Verification items for the finished model (mm, model axes). Coordinates: 2 decimals unless noted, no trailing zeros. Loops run counter-clockwise (first coordinate to the right, second up) from the corner with the lowest first, then second, coordinate; pieces in that order, holes last. Notation, with made-up numbers: (81, -7) -> (127, -7) arc R33 cw to (127, 23) -> close; hole circle Ø10 at (-6, -18.5). An arc over 180 degrees is marked (long way). Write item = value, one per line.
```python
from build123d import *

# Parameters (mm, degrees)
BOSS_EXTRUDE1_DEPTH = 6
SKETCH2_W           = 6
SKETCH2_H           = 37.5
CUT_EXTRUDE1_DEPTH  = 6
LPATTERN1_COUNT     = 4
LPATTERN1_PITCH     = 75
FILLET1_R           = 40
SKETCH3_W           = 6
SKETCH3_H           = 10
SKETCH3_H_2         = 112.5
CUT_EXTRUDE2_DEPTH  = 515.816472153
SKETCH4_W           = 15
SKETCH4_H           = 6
CUT_EXTRUDE3_DEPTH  = 515.816472153
SKETCH5_R           = 2
CUT_EXTRUDE4_DEPTH  = 515.816472153


with BuildPart() as part:
    # Sketch1 → Boss-Extrude1 (new body)
    with BuildSketch(Plane(origin=(0, 0, 0), x_dir=(0, 0, -1), z_dir=(1, 0, 0))):
        Polygon((450, 225), (450, 250), (0, 250), (0, 0), (450, 0), (450, 127.5), (30, 127.5), (30, 225), align=None)
    extrude(amount=BOSS_EXTRUDE1_DEPTH)

    # Sketch2 → Cut-Extrude1 (cut)
    with BuildSketch(Plane(origin=(6, 0, 0), x_dir=(0, 0, -1), z_dir=(1, 0, 0))):
        with Locations((3, 231.25)):
            Rectangle(SKETCH2_W, SKETCH2_H)
    cut_extrude1 = extrude(amount=-CUT_EXTRUDE1_DEPTH, mode=Mode.SUBTRACT)

    # LPattern1: Cut-Extrude1 ×4
    with Locations(*[(0, -i * LPATTERN1_PITCH, 0) for i in range(1, LPATTERN1_COUNT)]):
        add(cut_extrude1, mode=Mode.SUBTRACT)

    # Fillet1
    fillet1_edges = [part.edges().sort_by_distance(p)[0] for p in [
        (3, 225, -30),
    ]]
    fillet(fillet1_edges, radius=FILLET1_R)

    # Sketch3 → Cut-Extrude2 (cut, through all)
    with BuildSketch(Plane.ZY):
        with Locations((-447, 230)):
            Rectangle(SKETCH3_W, SKETCH3_H)
        with Locations((-447, 56.25)):
            Rectangle(SKETCH3_W, SKETCH3_H_2)
    extrude(amount=-CUT_EXTRUDE2_DEPTH, mode=Mode.SUBTRACT)

    # Sketch4 → Cut-Extrude3 (cut, through all)
    with BuildSketch(Plane.ZY):
        with Locations((-23.5, 3)):
            Rectangle(SKETCH4_W, SKETCH4_H)
        with Locations((-426.5, 3)):
            Rectangle(SKETCH4_W, SKETCH4_H)
    extrude(amount=-CUT_EXTRUDE3_DEPTH, mode=Mode.SUBTRACT)

    # Sketch5 → Cut-Extrude4 (cut, through all)
    with BuildSketch(Plane.ZY):
        with Locations((-384, 237.5)):
            Circle(SKETCH5_R)
        with Locations((-364, 237.5)):
            Circle(SKETCH5_R)
    extrude(amount=-CUT_EXTRUDE4_DEPTH, mode=Mode.SUBTRACT)


solid = part.part
```
1) Depth check by flat-ended pin: pin 1 Ø1.8 at (x, z) = (3, -2.5) entering from +Y; pin 2 Ø1.5 at (x, y) = (4.5, 161.5) entering from +Z; pin 3 Ø3 at (x, y) = (4.5, 4.5) entering from -Z; pin 4 Ø3.5 at (y, z) = (237.5, -364) entering from -X. Enter the tip coordinate at first touch or a pass-through.
Ans:
pin_1 = 212.5
pin_2 = -6
pin_3 = -444
pin_4 = through
2) Sectioned sample at C-C, the plane z = -44.5. Record the cut outline in (x, y), plus the area to 3 significant figures.
Ans:
outline = (0, 0) -> (6, 0) -> (6, 127.5) -> (0, 127.5) -> close; (0, 215.82) -> (6, 215.82) -> (6, 250) -> (0, 250) -> close
area = 970 mm2
3) Sectioned sample at A-A, the plane z = -177.5. Record the cut outline in (x, y).
Ans:
outline = (0, 0) -> (6, 0) -> (6, 127.5) -> (0, 127.5) -> close; (0, 225) -> (6, 225) -> (6, 250) -> (0, 250) -> close
4) Material ranges on line 1 (Y direction, x = 4.6, z = -364); line 2 (Z direction, x = 2.2, y = 237.5); line 3 (Y direction, x = 1.75, z = -224.5), recorded low to high.
Ans:
line_1 = 0 to 127.5, 225 to 235.5, 239.5 to 250
line_2 = -450 to -386, -382 to -366, -362 to -6
line_3 = 0 to 127.5, 225 to 250
5) Sectioned sample at D-D, the plane y = 164.5. Record the cut outline in (x, z), plus the area to 3 significant figures.
Ans:
outline = (0, -30) -> (6, -30) -> (6, -6) -> (0, -6) -> close
area = 144 mm2
6) Sectioned sample at B-B, the plane x = 2.75. Count the separate pieces of the cut face and the enclosed holes in it, plus the area to 3 significant figures.
Ans:
separate_pieces = 1
enclosed_holes = 2
area = 70,100 mm2
7) Release check for a two-part mould opening along Y. For faces 1 (the face through (3.042, 213.594, -42.028)), 2 (the face through (0, 99, -222)) record: pulls with the +Y half, pulls with the -Y half, needs draft (parallel to the pull), parting line crosses it, or undercut.
Ans:
face_1 = undercut
face_2 = needs draft
